Could you check a few things on this drawing? It's one solid part, dimensions in mm from its lowest x, y, z. A direction names the side the tool comes from. Give positions to 0.01 mm unless a question says otherwise; leave off trailing zeros. Write each loop counter-clockwise with the first axis right and the second up, starting at its lowest first coordinate (ties: lowest second). Pieces come first, ordered by that corner, then holes. Notation, with made-up numbers: (66, 8) -> (125, 8) arc R5 cw to (125, 12) -> close; hole circle Ø10 at (22, -9). An arc over 180 degrees is marked (long way). Use CSV: the item, a comma, the result in double quotes. Start each with the question number.
(1) Suppose I cut it at B-B on z = 25.6. List the corners of the cut face in (x, y) for me (1 decimal).
(2) Suppose I cut it at A-A on y = 18.3. List the corners of the cut face in (x, z) for me, plus the area to 3 significant figures.
(3) Suppose I cut it at D-D on x = 55. List the corners of the cut face in (y, z) for me.
(4) Suppose I cut it at C-C on x = 18. List the corners of the cut face in (y, z) for me, plus the area to 3 significant figures.
(5) For pin 1 Ø1.5 at (x, z) = (39, 30) entering from +Y; pin 2 Ø1.7 at (x, z) = (5.5, 26) entering from +Y; pin 3 Ø5 at (y, z) = (10.55, 31.72) entering from -X, each with a flat end and sliding along its axis, tell me the tip position at first contact or that it passes through.
(6) Which directions (+Z, -Z, +X, -X, +Y, -Y) give clear straight access to the entire face, cutting with the end or side of a thin tool? Please do the marked faces 1, 2 and 3.
(7) I need wall thicknesses on L1, parallel to Y at x = 26, z = 18; L2, parallel to X at y = 20, z = 19; L3, parallel to X at y = 10.5, z = 12. Which ranges of each line are inside material? Lowest first, please. Write a range as [from, to].
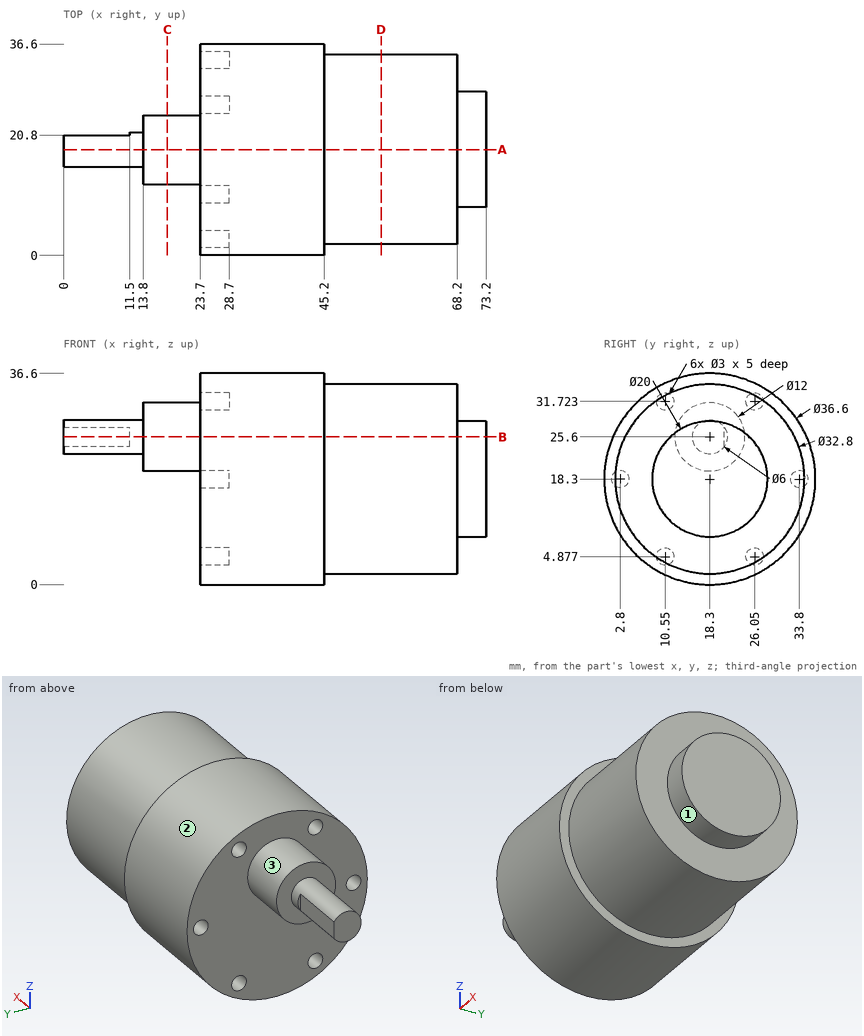
Geometry says:
1,outline,"(0, 15.3) -> (13.8, 15.3) -> (13.8, 12.3) -> (23.7, 12.3) -> (23.7, 1.5) -> (45.2, 1.5) -> (45.2, 3.6) -> (68.2, 3.6) -> (68.2, 11.5) -> (73.2, 11.5) -> (73.2, 25.1) -> (68.2, 25.1) -> (68.2, 33) -> (45.2, 33) -> (45.2, 35.1) -> (23.7, 35.1) -> (23.7, 24.3) -> (13.8, 24.3) -> (13.8, 21.3) -> (11.5, 21.3) -> (11.5, 20.8) -> (0, 20.8) -> close"
2,outline,"(0, 22.6) -> (13.8, 22.6) -> (13.8, 19.6) -> (23.7, 19.6) -> (23.7, 0) -> (45.2, 0) -> (45.2, 1.9) -> (68.2, 1.9) -> (68.2, 8.3) -> (73.2, 8.3) -> (73.2, 28.3) -> (68.2, 28.3) -> (68.2, 34.7) -> (45.2, 34.7) -> (45.2, 36.6) -> (23.7, 36.6) -> (23.7, 31.6) -> (13.8, 31.6) -> (13.8, 28.6) -> (0, 28.6) -> close"
2,area,"1,840 mm²"
3,outline,"circle Ø32.8 at (18.3, 18.3)"
4,outline,"circle Ø12 at (18.3, 25.6)"
4,area,"113 mm²"
5,pin 1,"y = 32.96"
5,pin 2,"y = 20.8"
5,pin 3,"x = 23.7"
6,face 1,"+X"
6,face 2,"+X, -X"
6,face 3,"-X"
7,L1,"[0, 1.33], [4.27, 32.33], [35.27, 36.6]"
7,L2,"[23.7, 73.2]"
7,L3,"[23.7, 68.2]"
